Geometry check sheet. Reference: the model listing, model coordinates, mm. Face numbers are marked on the shaded views. A direction names the side the tool comes from. Round coordinates to 2 decimals unless told otherwise and drop trailing zeros. Order: outer loops, then holes, each group sorted by start corner. A loop starts at its lowest first (then second) coordinate and runs counter-clockwise, first axis right, second up. Notation, with made-up numbers: M 43,34 L 90,34 A14 ccw 90,59 Z; hole C 63.5,76.5 d5. An arc over 180 degrees is marked long. Return JSON: item names as keys, results as strings. Group by question number.
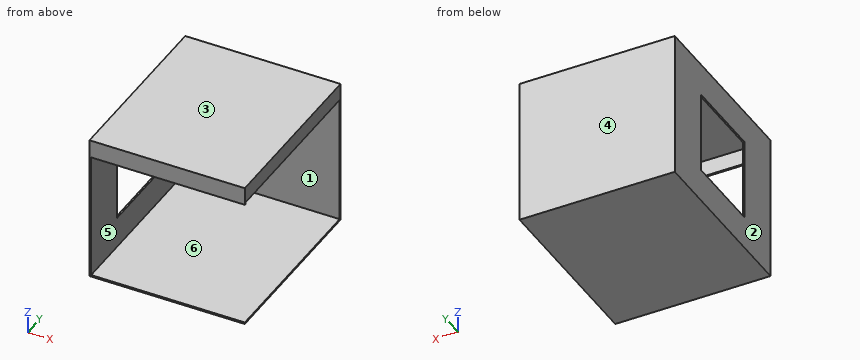
```python
from build123d import *

# Parameters (mm, degrees)
F0_W     = 241.3
F0_H     = 279.4
F1_DEPTH = 228.6
F2_T     = -2.54
F3_W     = 127
F3_H     = 127
F4_DEPTH = 25.4
F5_W     = 276.86
F5_H     = 200.66
F6_DEPTH = 25.4
F7_W     = 2.54
F7_H     = 25.4
F8_DEPTH = 238.76


with BuildPart() as f1:
    # F0 (on Top) → F1 (new body)
    with BuildSketch(Plane.XY):
        Rectangle(F0_W, F0_H)
    extrude(amount=F1_DEPTH)

    # F2
    f2_openings = [f1.faces().sort_by_distance(p)[0] for p in [
        (0, -139.7, 114.3),
    ]]
    offset(amount=F2_T, openings=f2_openings)

    # F3 (on face) → F4 (cut)
    with BuildSketch(Plane.YZ.offset(-118.11)):
        with Locations((0, 114.533028)):
            Rectangle(F3_W, F3_H)
    extrude(amount=-F4_DEPTH, mode=Mode.SUBTRACT)

    # F5 (on face) → F6 (cut)
    with BuildSketch(Plane.YZ.offset(120.65)):
        with Locations((-1.27, 102.87)):
            Rectangle(F5_W, F5_H)
    extrude(amount=-F6_DEPTH, mode=Mode.SUBTRACT)

    # F7 (on face) → F8 (join, through all)
    with BuildSketch(Plane.YZ.offset(-118.11)):
        with Locations((-138.43, 213.36)):
            Rectangle(F7_W, F7_H)
    extrude(amount=F8_DEPTH)


solid = f1.part
```
Q1. Section check C-C on x = 52. Record the cut outline in (y, z).
Q2. Release check for a two-part mould opening along Z. For the marked faces 1, 2 and 3 record: +Z half, -Z half, draft (parallel to the pull), parting line (faces both ways), or undercut.
Q3. Section check B-B on z = 133. Record the cut outline in (x, y).
Q4. Set-up check for the marked faces 4, 5 and 6: record each of +Z, -Z, +X, -X, +Y, -Y from which the full face is reachable in a straight line by a thin tool's end or side.
Q5. Depth check by flat-ended pin: pin 1 Ø2 at (x, z) = (-77, 195) entering from -Y. Enter the tip coordinate at first touch or a pass-through.
Q6. Material ranges on line 1 along Z through (x, y) = (-18, 72); line 2 along X through (y, z) = (-107, 211); line 3 along Y through (x, z) = (-76, 203), recorded low to high.
Q7. Section check A-A on y = 40.5. Record the cut outline in (x, z).
Q8. Section check D-D on y = 117. Record the cut outline in (x, z), plus the area to 3 significant figures.
Geometry check:
{
 "1": {"outline": "M -139.7,0 L 139.7,0 L 139.7,228.6 L -139.7,228.6 L -139.7,200.66 L -137.16,200.66 L -137.16,226.06 L 137.16,226.06 L 137.16,2.54 L -139.7,2.54 Z"},
 "2": {"face 1": "undercut", "face 2": "draft", "face 3": "+Z half"},
 "3": {"outline": "M -120.65,-139.7 L -118.11,-139.7 L -118.11,-63.5 L -120.65,-63.5 Z; M -120.65,63.5 L -118.11,63.5 L -118.11,137.16 L 120.65,137.16 L 120.65,139.7 L -120.65,139.7 Z"},
 "4": {"face 4": "+Z, -Z, +X, -X, +Y", "face 5": "none", "face 6": "+X, -Y"},
 "5": {"pin 1": "stops at y = 137.16"},
 "6": {"line 1": "z = 0 to 2.54, 226.06 to 228.6", "line 2": "x = -120.65 to -118.11, 118.11 to 120.65", "line 3": "y = -139.7 to -137.16, 137.16 to 139.7"},
 "7": {"outline": "M -120.65,0 L 120.65,0 L 120.65,2.54 L -118.11,2.54 L -118.11,51.03 L -120.65,51.03 Z; M -120.65,178.03 L -118.11,178.03 L -118.11,226.06 L 118.11,226.06 L 118.11,203.2 L 120.65,203.2 L 120.65,228.6 L -120.65,228.6 Z"},
 "8": {"outline": "M -120.65,0 L 120.65,0 L 120.65,2.54 L -118.11,2.54 L -118.11,226.06 L 118.11,226.06 L 118.11,203.2 L 120.65,203.2 L 120.65,228.6 L -120.65,228.6 Z", "area": "1,850 mm^2"}
}
